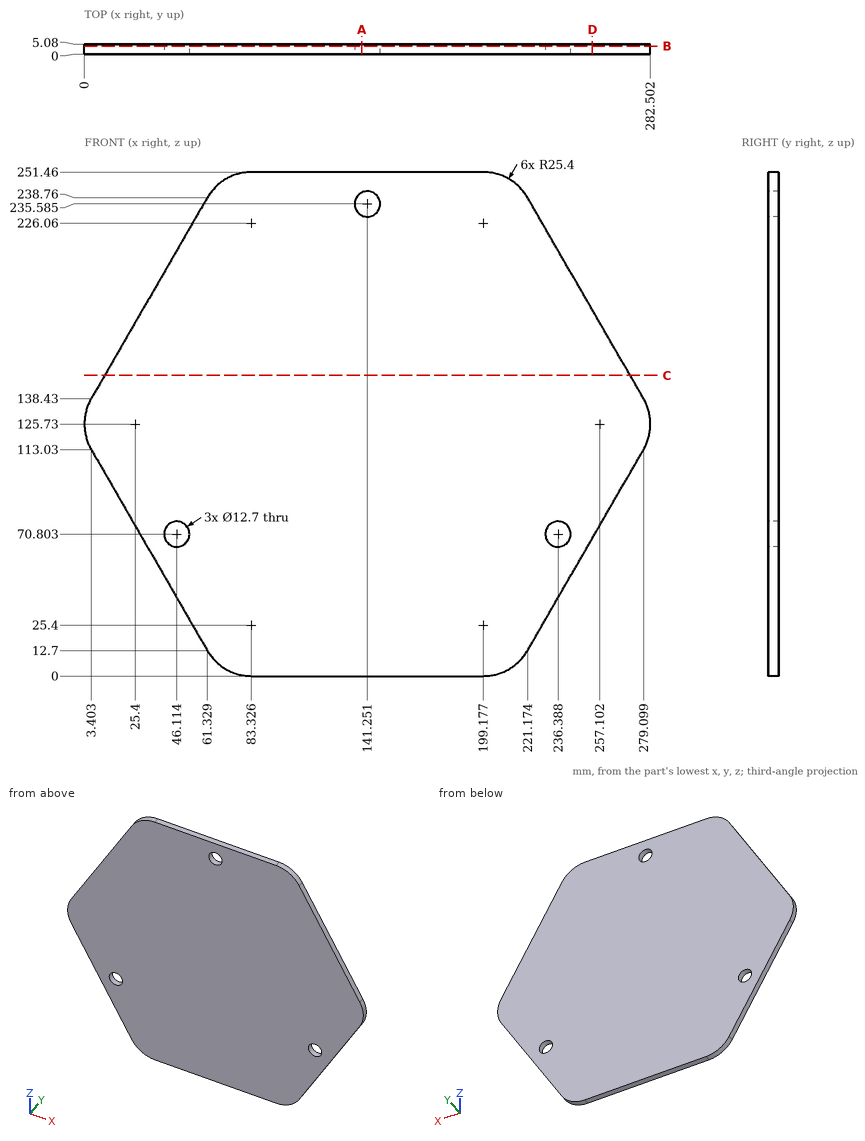
Job drawing, mm, ordinate dimensions from the low corner. One solid piece. Coordinates: 2 decimals unless noted, no trailing zeros. Order: outer loops, then holes, each group sorted by start corner. A loop starts at its lowest first (then second) coordinate and runs counter-clockwise, first axis right, second up. Notation, with made-up numbers: (78, 18.5) -> (119, 18.5) arc R20 cw to (119, 33.5) -> close; hole circle Ø4 at (55, -27). An arc over 180 degrees is marked (long way). Answer in a Markdown table with one row per item. Add a question column.
Q1. Drop flat-ended pins along their axis: pin 1 (2 mm diameter, centred on y = 2.5, z = 82.5, fed in from -X); pin 2 (11.5 mm diameter, centred on x = 46.11, z = 70.8, fed in from +Y); pin 3 (3 mm diameter, centred on y = 2, z = 204.5, fed in from -X). Give the stop position or say it passes through.
Q2. Band-saw the part on D-D, the plane x = 253.5. List the corners of the cut face in (y, z).
Q3. Band-saw the part on C-C, the plane z = 150. List the corners of the cut face in (x, y).
Q4. Wall check: line 1 along X through (y, z) = (0.25, 67.5) (1 decimal); line 2 along Z through (x, y) = (82, 2.9) (1 decimal); line 3 along X through (y, z) = (3.5, 115.5). Give the ranges that are in metal, low to high. Write a range as [from, to].
Q5. Band-saw the part on A-A, the plane x = 138.5. List the corners of the cut face in (y, z), then the cut area to 3 significant figures.
Q6. Band-saw the part on B-B, the plane y = 4.05. Give the number of separate pieces and of enclosed holes in the cut face, then the cut area to 3 significant figures.
Answers follow:
| question | item | result |
|---|---|---|
| 1 | pin 1 | x = 20.45 |
| 1 | pin 2 | through |
| 1 | pin 3 | x = 40.68 |
| 2 | outline | (0, 68.69) -> (5.08, 68.69) -> (5.08, 182.77) -> (0, 182.77) -> close |
| 3 | outline | (10.08, 0) -> (272.42, 0) -> (272.42, 5.08) -> (10.08, 5.08) -> close |
| 4 | line 1 | [29.7, 40.7], [51.5, 231], [241.8, 252.8] |
| 4 | line 2 | [0, 251.4] |
| 4 | line 3 | [2.15, 280.35] |
| 5 | outline | (0, 0) -> (5.08, 0) -> (5.08, 229.86) -> (0, 229.86) -> close; (0, 241.31) -> (5.08, 241.31) -> (5.08, 251.46) -> (0, 251.46) -> close |
| 5 | area | 1,220 mm^2 |
| 6 | separate pieces | 1 |
| 6 | enclosed holes | 3 |
| 6 | area | 54,200 mm^2 |
